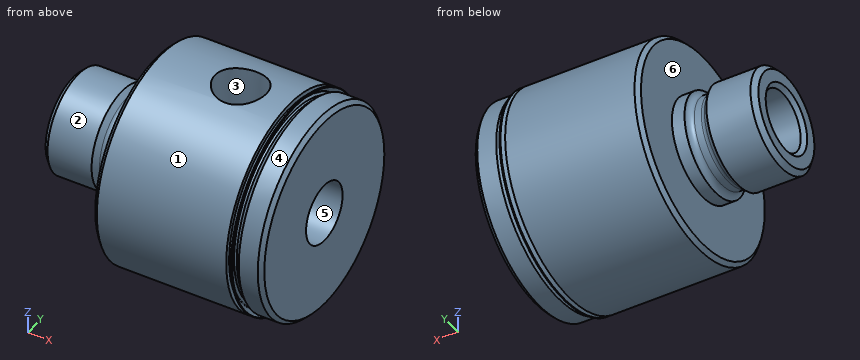
Autodesk Inventor part; units mm, degrees
ref_plane "dp1_XY" through (15.875, 9.4932, 0) normal (0, 0, 1) x (1, 0, 0)
ref_plane "dp1_YZ" through (15.875, 9.4932, 0) normal (1, 0, 0) x (0, 1, 0)
ref_plane "dp1_ZX" through (15.875, 9.4932, 0) normal (0, 1, 0) x (0, 0, 1)
sketch "Sketch_2" plane through (0, 0, 0) normal (0, 0, 1) x (1, 0, 0)
  line L0 (15.875, 0) -> (0, 0)
  line L1 (0, 0) -> (0, 8.589)
  line L2 (0, 8.589) -> (0.936, 9.525)
  line L3 (0.936, 9.525) -> (9.31, 9.525)
  line L4 (9.31, 9.525) -> (10.2623, 8.6108)
  arc A0 (10.2623, 8.6108) -> (11.0363, 8.2995) centre (11.0363, 9.417) ccw
  line L5 (11.0363, 8.2995) -> (12.3698, 8.2995)
  arc A1 (12.3698, 8.2995) -> (13.4874, 9.417) centre (12.3698, 9.4171) ccw
  line L6 (13.4874, 9.417) -> (13.4874, 9.4932)
  line L7 (13.4874, 9.4932) -> (15.875, 9.4932)
  line L8 (15.875, 9.4932) -> (15.875, 0)
  line L9 (15.875, 0) -> (0, 0)
revolve "Revolution1" add sketch "Sketch_2" angle 360 about axis through (15.875, 0, 0) along (1, 0, 0)
thread "Thread1"
sketch "Sketch_3" plane through (0, 0, 0) normal (0, 0, 1) x (1, 0, 0)
  line L0 (47.625, 0) -> (15.875, 0)
  line L1 (15.875, 0) -> (15.875, 19.0055)
  line L2 (15.875, 19.0055) -> (16.637, 19.7675)
  line L3 (16.637, 19.7675) -> (41.2115, 19.7675)
  line L4 (41.2115, 19.7675) -> (41.2115, 18.1801)
  line L5 (41.2115, 18.1801) -> (42.2275, 18.1801)
  line L6 (42.2275, 18.1801) -> (43.2435, 19.196)
  line L7 (43.2435, 19.196) -> (46.863, 19.196)
  line L8 (46.863, 19.196) -> (47.625, 18.434)
  line L9 (47.625, 18.434) -> (47.625, 0)
  line L10 (47.625, 0) -> (15.875, 0)
revolve "Revolution2" add sketch "Sketch_3" angle 360 about axis through (47.625, 0, 0) along (1, 0, 0)
sketch "Sketch3" plane through (0, 0, 0) normal (-1, 0, 0) x (0, 0, 1)
  point P0 (0, 0)
hole "Hole1" at (0, 0, 0) direction (1, 0, 0) diameter 11.2268 depth 47.625 countersink diameter 12.7508 countersink angle 90
sketch "Sketch_40" plane through (0, 0, 0) normal (0, 1, 0) x (-1, 0, 0)
  line L0 (-31.75, 19.7675) -> (-31.75, 0)
  line L1 (-31.75, 0) -> (-34.925, 0)
  line L2 (-34.925, 0) -> (-34.925, 7.7681)
  line L3 (-34.925, 7.7681) -> (-36.2564, 9.0996)
  line L4 (-36.2564, 9.0996) -> (-36.5895, 19.7675)
  line L5 (-36.5895, 19.7675) -> (-31.75, 19.7675)
  line L6 (-31.75, 19.7675) -> (-31.75, 0)
revolve "Revolution3" cut sketch "Sketch_40" angle 360 about axis through (31.75, 0, 19.7675) along (0, 0, 1)
thread "Thread2"
sketch "Sketch_47" plane through (0, 0, 0) normal (0, 0, 1) x (1, 0, 0)
  line L0 (42.2275, 0) -> (41.2115, 0)
  line L1 (41.2115, 18.8883) -> (41.2115, 17.9261)
  line L2 (41.2115, 17.9261) -> (42.2275, 17.9261)
  line L3 (42.2275, 17.9261) -> (42.2275, 18.1801)
  line L4 (42.2275, 18.1801) -> (41.7195, 18.1801)
  line L5 (41.7195, 18.1801) -> (41.3449, 18.5547)
  arc A0 (41.3449, 18.7343) -> (41.3449, 18.5547) centre (41.4347, 18.6445) ccw
  line L6 (41.3449, 18.7343) -> (42.294, 19.6834)
  line L7 (42.294, 19.6834) -> (42.294, 19.7675)
  line L8 (42.294, 19.7675) -> (42.0908, 19.7675)
  line L9 (42.0908, 19.7675) -> (41.2115, 18.8883)
revolve "Revolution4" add sketch "Sketch_47" angle 360 about axis through (42.2275, 0, 0) along (1, 0, 0)
ref_plane "dp1_XY" through (15.875, 9.4932, 0) normal (0, 0, 1) x (1, 0, 0)
ref_plane "dp1_YZ" through (15.875, 9.4932, 0) normal (1, 0, 0) x (0, 1, 0)
ref_plane "dp1_ZX" through (15.875, 9.4932, 0) normal (0, 1, 0) x (0, 0, 1)
ref_plane "dp2_XY" through (15.875, -9.4932, 0) normal (0, 0, 1) x (1, 0, 0)
ref_plane "dp2_YZ" through (15.875, -9.4932, 0) normal (1, 0, 0) x (0, 1, 0)
ref_plane "dp2_ZX" through (15.875, -9.4932, 0) normal (0, 1, 0) x (0, 0, 1)
ref_plane "hh_XY" through (0, 9.525, 0) normal (0, 0, 1) x (1, 0, 0)
ref_plane "hh_YZ" through (0, 9.525, 0) normal (1, 0, 0) x (0, 1, 0)
ref_plane "hh_ZX" through (0, 9.525, 0) normal (0, 1, 0) x (0, 0, 1)
ref_plane "port_XY" through (31.75, 0, 0) normal (0, 0, 1) x (1, 0, 0)
ref_plane "port_YZ" through (31.75, 0, 0) normal (1, 0, 0) x (0, 1, 0)
ref_plane "port_ZX" through (31.75, 0, 0) normal (0, 1, 0) x (0, 0, 1)
ref_plane "rod_guide_XY" through (0, 0, 0) normal (1, 0, 0) x (0, 0, -1)
ref_plane "rod_guide_YZ" through (0, 0, 0) normal (0, 0, -1) x (0, 1, 0)
ref_plane "rod_guide_ZX" through (0, 0, 0) normal (0, 1, 0) x (1, 0, 0)
ref_plane "s1_XY" through (13.4874, 0, 0) normal (0, 0, 1) x (1, 0, 0)
ref_plane "s1_YZ" through (13.4874, 0, 0) normal (1, 0, 0) x (0, 1, 0)
ref_plane "s1_ZX" through (13.4874, 0, 0) normal (0, 1, 0) x (0, 0, 1)
ref_plane "s2_XY" through (15.875, 0, 0) normal (0, 0, 1) x (1, 0, 0)
ref_plane "s2_YZ" through (15.875, 0, 0) normal (1, 0, 0) x (0, 1, 0)
ref_plane "s2_ZX" through (15.875, 0, 0) normal (0, 1, 0) x (0, 0, 1)
ref_plane "t1_XY" through (15.875, 0, 0) normal (1, 0, 0) x (0, 0, -1)
ref_plane "t1_YZ" through (15.875, 0, 0) normal (0, 0, -1) x (0, 1, 0)
ref_plane "t1_ZX" through (15.875, 0, 0) normal (0, 1, 0) x (1, 0, 0)
ref_plane "t111_XY" through (15.875, 0, 0) normal (1, 0, 0) x (0, 0, -1)
ref_plane "t111_YZ" through (15.875, 0, 0) normal (0, 0, -1) x (0, 1, 0)
ref_plane "t111_ZX" through (15.875, 0, 0) normal (0, 1, 0) x (1, 0, 0)
ref_plane "to_foot_bracket_XY" through (15.875, 0, 0) normal (1, 0, 0) x (0, 0, -1)
ref_plane "to_foot_bracket_YZ" through (15.875, 0, 0) normal (0, 0, -1) x (0, 1, 0)
ref_plane "to_foot_bracket_ZX" through (15.875, 0, 0) normal (0, 1, 0) x (1, 0, 0)
ref_plane "to_nut_XY" through (13.4874, 0, 0) normal (1, 0, 0) x (0, 0, -1)
ref_plane "to_nut_YZ" through (13.4874, 0, 0) normal (0, 0, -1) x (0, 1, 0)
ref_plane "to_nut_ZX" through (13.4874, 0, 0) normal (0, 1, 0) x (1, 0, 0)
ref_plane "to_rod_XY" through (-127, 0, 0) normal (1, 0, 0) x (0, 0, -1)
ref_plane "to_rod_YZ" through (-127, 0, 0) normal (0, 0, -1) x (0, 1, 0)
ref_plane "to_rod_ZX" through (-127, 0, 0) normal (0, 1, 0) x (1, 0, 0)
ref_plane "to_screw_XY" through (31.75, 14.2875, -10.0711) normal (0, 1, 0) x (1, 0, 0)
ref_plane "to_screw_YZ" through (31.75, 14.2875, -10.0711) normal (1, 0, 0) x (0, 0, -1)
ref_plane "to_screw_ZX" through (31.75, 14.2875, -10.0711) normal (0, 0, -1) x (0, 1, 0)
ref_plane "to_trunnion_brackets_XY" through (26.9494, 0, 0) normal (0, 1, 0) x (1, 0, 0)
ref_plane "to_trunnion_brackets_YZ" through (26.9494, 0, 0) normal (1, 0, 0) x (0, 0, -1)
ref_plane "to_trunnion_brackets_ZX" through (26.9494, 0, 0) normal (0, 0, -1) x (0, 1, 0)
ref_plane "to_trunnion_brackets1_XY" through (26.9494, 22.225, 0) normal (0, 1, 0) x (1, 0, 0)
ref_plane "to_trunnion_brackets1_YZ" through (26.9494, 22.225, 0) normal (1, 0, 0) x (0, 0, -1)
ref_plane "to_trunnion_brackets1_ZX" through (26.9494, 22.225, 0) normal (0, 0, -1) x (0, 1, 0)
ref_plane "to_trunnion_brackets2_XY" through (26.9494, -22.225, 0) normal (0, 1, 0) x (1, 0, 0)
ref_plane "to_trunnion_brackets2_YZ" through (26.9494, -22.225, 0) normal (1, 0, 0) x (0, 0, -1)
ref_plane "to_trunnion_brackets2_ZX" through (26.9494, -22.225, 0) normal (0, 0, -1) x (0, 1, 0)
ref_plane "to_tube_XY" through (42.2275, 0, 0) normal (1, 0, 0) x (0, 0, -1)
ref_plane "to_tube_YZ" through (42.2275, 0, 0) normal (0, 0, -1) x (0, 1, 0)
ref_plane "to_tube_ZX" through (42.2275, 0, 0) normal (0, 1, 0) x (1, 0, 0)
properties part number "17R000-5_rod_guide" material "Aluminum 6061"
Build history of the part. All positions in model axes, mm. Face numbers are marked on the shaded views. A direction names the side the tool comes from. Give positions to 0.01 mm unless a question says otherwise; leave off trailing zeros. Loops run counter-clockwise (first coordinate to the right, second up) from the corner with the lowest first, then second, coordinate; pieces in that order, holes last.
Item 1: Slice it at C-C, the plane x = 31.75. List the corners of the cut face in (y, z) (1 decimal), and give its area (3 significant figures).
Answers follow:
outline: (-4.8, 19.2) arc R19.8 ccw (long way) to (4.8, 19.2) - (4.5, 9.1) - (3.2, 7.8) - (3.2, 4.6) arc R5.6 cw (long way) to (-3.2, 4.6) - (-3.2, 7.8) - (-4.5, 9.1) - close
area: 1,000 mm2
Item 2: Slice it at D-D, the plane x = 24. List the corners of the cut face in (y, z) (1 decimal).
Answers follow:
outline: circle Ø39.5 at (0, 0); hole circle Ø11.2 at (0, 0)
Item 3: Pull direction Y, two halves, no side cores. Call the marked faces 4, 5 and 6: released by +Y, released by -Y, zero draft, split by the parting line, or undercut.
Answers follow:
face 4: split by the parting line
face 5: undercut
face 6: zero draft
Item 4: Which spindle directions (+Z, -Z, +X, -X, +Y, -Y) get a long thin tool onto all of the face, cutting with end or side? Do the marked faces 1, 2 and 3. Say none if no direction does.
Answers follow:
face 1: +X, -X
face 2: -X
face 3: +Z
Item 5: Flat gauge pins, fed straight in: pin 1 (4 mm diameter, centred on x = 35.5, z = -14, fed in from -Y); pin 2 (12 mm diameter, centred on y = -15, z = -13, fed in from -X) (3 decimals); pin 3 (12 mm diameter, centred on x = 14, y = 11.5, fed in from -Z); pin 4 (3 mm diameter, centred on x = 11.5, z = -11.5, fed in from +Y). Where does each tip first touch, or does it go through?
Answers follow:
pin 1: stops at y = -15.71
pin 2: stops at x = 15.875
pin 3: stops at z = -18.8
pin 4: passes through
Item 6: Slice it at B-B, the plane y = 0. Give the number of separate pieces and of enclosed holes in the cut face, and give its area (3 significant figures).
Answers follow:
separate pieces: 3
enclosed holes: 0
area: 879 mm2
Item 7: Drill centre lines: line 1 (X direction, y = 0, z = 6.6) (3 decimals); line 2 (Y direction, x = 23, z = -2); line 3 (X direction, y = -15.5, z = 7.5) (3 decimals). Where is each one in solid material? Low to high.
Answers follow:
line 1: x = 0 to 28.575, 34.925 to 47.625
line 2: y = -19.67 to -5.25, 5.25 to 19.67
line 3: x = 15.875 to 47.625
Item 8: Slice it at A-A, the plane x = 45.5. List the corners of the cut face in (y, z), and give its area (3 significant figures).
Answers follow:
outline: circle Ø38.39 at (0, 0); hole circle Ø11.23 at (0, 0)
area: 1,060 mm2
